CAD build for the part. Positions are in the model's coordinates, mm. A direction names the side the tool comes from. Round coordinates to 2 decimals unless told otherwise and drop trailing zeros. Write each loop counter-clockwise with the first axis right and the second up, starting at its lowest first coordinate (ties: lowest second). Pieces come first, ordered by that corner, then holes. Notation, with made-up numbers: (-4, 76) - (24, 76) arc R20 ccw to (24, 92) - close; hole circle Ø7 at (28, 65). An arc over 180 degrees is marked (long way). Put each result on its own line as item: value. Start each with the question number.
Item 1: Cut at B-B (y = 6). Give the cut face in (x, z), and give its area (3 significant figures).
Item 2: Cut at D-D (x = 6.5). Give the cut face in (y, z).
Item 3: Cut at A-A (x = 36). Give the cut face in (y, z).
Item 4: Pin check, flat tips, straight feed: pin 1 Ø5 at (x, y) = (68.5, 6.5) entering from +Z; pin 2 Ø1.5 at (x, z) = (48.5, -26) entering from -Y; pin 3 Ø11 at (x, z) = (30.5, -13) entering from +Y; pin 4 Ø13 at (x, z) = (5.5, -11) entering from +Y. Stop position of each tip, or through.
Item 5: 3-axis set-ups, long thin cutter, end or side, ignore diameter. For faces 1 (the flat face through (42, 12, -22)), 2 (the flat face through (6, 20, -18)), 3 (the flat face through (67, 6, -20)), 4 (the flat face through (31, 6, 0)), 5 (the flat face through (72, 6, -28)): which of +Z, -Z, +X, -X, +Y, -Y reach the whole face in a straight line?
Item 6: Drill centre lines: line 1 (X direction, y = 9, z = -18); line 2 (Y direction, x = 46, z = -5.5); line 3 (Z direction, x = 34, y = 5). Where is each one in solid material? Low to high. Write a range as from..to.
Item 7: Cut at C-C (z = -9). Give the cut face in (x, y), and give its area (3 significant figures).
Item 8: Mould opens along X. For faces 6 (the cylindrical face through (42.94, 5.92, -18.91)), 7 (the flat face through (27, 9, -36)), 8 (the flat face through (0, 9, -18)), 9 (the flat face through (62, 6, -10)) say: released by +X, released by -X, zero draft, split by the parting line, or undercut.
```python
from build123d import *

# Parameters (mm, degrees)
SKETCH_1_R      = 7
EXTRUDE_1_DEPTH = 12
SKETCH_2_W      = 12
SKETCH_2_H      = 18
EXTRUDE_2_DEPTH = 4
SKETCH_3_W      = 12
SKETCH_3_H      = 18
EXTRUDE_3_DEPTH = 12


with BuildPart() as part:
    # 草圖1 → 填料-伸長1 (new body)
    with BuildSketch(Plane(origin=(0, 0, 0), x_dir=(1, 0, 0), z_dir=(0, 1, 0))):
        Polygon((0, 0), (62, 0), (62, 20), (72, 20), (72, 36), (0, 36), align=None)
        with Locations(Location((36, 18, 0), (0, 0, 270))):
            Circle(SKETCH_1_R, mode=Mode.SUBTRACT)
    extrude(amount=EXTRUDE_1_DEPTH)

    # 草圖2 → 填料-伸長2 (add)
    with BuildSketch(Plane(origin=(0, 12, 0), x_dir=(1, 0, 0), z_dir=(0, 1, 0))):
        with Locations((6, 9)):
            Rectangle(SKETCH_2_W, SKETCH_2_H)
    extrude(amount=EXTRUDE_2_DEPTH)

    # 草圖3 → 填料-伸長3 (add)
    with BuildSketch(Plane(origin=(0, 12, 0), x_dir=(1, 0, 0), z_dir=(0, 1, 0))):
        with Locations((6, 27)):
            Rectangle(SKETCH_3_W, SKETCH_3_H)
    extrude(amount=EXTRUDE_3_DEPTH)


solid = part.part
```
Output values:
1. outline: (0, -36) - (72, -36) - (72, -20) - (62, -20) - (62, 0) - (0, 0) - close; hole circle Ø14 at (36, -18)
1. area: 2,240 mm2
2. outline: (0, -36) - (24, -36) - (24, -18) - (16, -18) - (16, 0) - (0, 0) - close
3. outline: (0, -36) - (12, -36) - (12, -25) - (0, -25) - close; (0, -11) - (12, -11) - (12, 0) - (0, 0) - close
4. pin 1: z = -20
4. pin 2: y = 0
4. pin 3: y = 12
4. pin 4: y = 16
5. face 1: +Z, -Z, +X, +Y
5. face 2: +Z, +X, -X, +Y
5. face 3: +Z, +X, +Y, -Y
5. face 4: +Z, +X, -X, +Y, -Y
5. face 5: +Z, -Z, +X, +Y, -Y
6. line 1: 0..29, 43..62
6. line 2: 0..12
6. line 3: -36..-24.71, -11.29..0
7. outline: (0, 0) - (62, 0) - (62, 12) - (12, 12) - (12, 16) - (0, 16) - close
7. area: 792 mm2
8. face 6: undercut
8. face 7: zero draft
8. face 8: released by -X
8. face 9: released by +X
